Input: part model. Units: mm. Frame: model coordinates. A direction names the side the tool comes from. Coordinates: 2 decimals unless noted, no trailing zeros.
Item 1: Reachability of faces 5 (the flat face through (-62, 0, -33)), 6 (the flat face through (-70, 5, -32)) from +Z, -Z, +X, -X, +Y, -Y: full face, straight path, thin tool, end or side. Return the list, or none.
Item 2: Ray query, line 1 along X through (y, z) = (6.5, -19.5); line 2 along X through (y, z) = (7.25, -30); line 3 along Z through (x, y) = (-68.5, 9.25). Return the intervals inside material, ascending.
Item 3: Contact query for flat-ended pins moving along their axis: P1, Ø0.5, axis at x = -81.5, y = 8.5, coming from the -Z side; P2, Ø1.5, axis at y = 7, z = -29.5, coming from the -X side; P3, Ø1.5, axis at y = 2.5, z = -27.5, coming from the +X side. Output: stop coordinate, or through.
Item 4: Pull-direction query (Z, two-part tool) for faces 1 (the flat face through (-62, 10, -32)), 2 (the flat face through (-82, 9, -31.447)), 3 (the flat face through (-66.417, 8, -32)), 4 (the flat face through (-58.417, 8, -32)); classes: released by +Z, released by -Z, zero draft, split by the parting line, or undercut.
```python
from build123d import *

# Parameters (mm, degrees)
SKETCH1_R           = 20
BOSS_EXTRUDE1_DEPTH = 10
THREAD1_PITCH       = 3.175
CUT_EXTRUDE2_DEPTH  = 5


with BuildPart() as part:
    # Sketch1 → Boss-Extrude1 (new body)
    with BuildSketch(Plane(origin=(0, 0, 0), x_dir=(1, 0, 0), z_dir=(0, 1, 0))):
        with Locations(Location((-62.417227704, 31.446847546, 0), (0, 0, 270))):
            Circle(SKETCH1_R)
    extrude(amount=BOSS_EXTRUDE1_DEPTH)

    # Thread1: the profile of Thread Profile1 profile screwed along a right-hand helix of 3.149606 turns, 12 arcs to a turn; built about Z, then put on its axis
    thread1_z = Axis((0, 0, 0), (0, 0, 1))
    thread1_corners = [(20.0003, 0, -0.000173205), (20.0003, 0, 2.778298196), (18.281480847, 0, 1.785937496), (18.281480847, 0, 0.992187496)]
    with BuildLine(mode=Mode.PRIVATE) as thread1_profile:
        Line(thread1_corners[0], thread1_corners[1])
        Line(thread1_corners[1], thread1_corners[2])
        Line(thread1_corners[2], thread1_corners[3])
        Line(thread1_corners[3], thread1_corners[0])
    thread1_cap = Face(thread1_profile.wire())
    thread1_turn_angles = [0, 15, 30, 45, 60, 75, 90, 105, 120, 135, 150, 165, 180, 195, 210, 225, 240, 255, 270, 285, 300, 315, 330, 345, 360]
    thread1_turn_weights = [1, 0.9659258262890683, 1, 0.9659258262890683, 1, 0.9659258262890683, 1, 0.9659258262890683, 1, 0.9659258262890683, 1, 0.9659258262890683, 1, 0.9659258262890683, 1, 0.9659258262890683, 1, 0.9659258262890683, 1, 0.9659258262890683, 1, 0.9659258262890683, 1, 0.9659258262890683, 1]
    thread1_turn_rails = [Edge.make_bspline([Vector(p[0], p[1], 0).rotate(thread1_z, thread1_turn_angles[k]) / thread1_turn_weights[k] + Vector(0, 0, p[2] + THREAD1_PITCH * thread1_turn_angles[k] / 360) for k in range(25)], [0, 0, 0, 1, 1, 2, 2, 3, 3, 4, 4, 5, 5, 6, 6, 7, 7, 8, 8, 9, 9, 10, 10, 11, 11, 12, 12, 12], 2, thread1_turn_weights) for p in thread1_corners]
    thread1_turn_sides = [Face.make_surface_from_curves(thread1_turn_rails[p[0]], thread1_turn_rails[p[1]]) for p in [(0, 1), (1, 2), (2, 3), (3, 0)]]
    thread1_last_angles = [1080, 1095, 1110, 1121.929133858, 1133.858267717]
    thread1_last_weights = [1, 0.9659258262890683, 1, 0.9784040075425771, 1]
    thread1_last_rails = [Edge.make_bspline([Vector(p[0], p[1], 0).rotate(thread1_z, thread1_last_angles[k]) / thread1_last_weights[k] + Vector(0, 0, p[2] + THREAD1_PITCH * thread1_last_angles[k] / 360) for k in range(5)], [0, 0, 0, 1, 1, 2, 2, 2], 2, thread1_last_weights) for p in thread1_corners]
    thread1_last_sides = [Face.make_surface_from_curves(thread1_last_rails[p[0]], thread1_last_rails[p[1]]) for p in [(0, 1), (1, 2), (2, 3), (3, 0)]]
    thread1 = Plane(origin=(-62.417227704, 10, -31.446847546), x_dir=(-1, 0, 0), z_dir=(0, -1, 0)) * Solid(Shell([*[p.moved(Location((0, 0, THREAD1_PITCH * i))) for i in range(3) for p in thread1_turn_sides], *thread1_last_sides, thread1_cap, thread1_cap.rotate(thread1_z, 1133.858267717).moved(Location((0, 0, THREAD1_PITCH * 1133.858267717 / 360)))]))
    add(thread1, mode=Mode.SUBTRACT)

    # Sketch9 → Cut-Extrude2 (cut)
    with BuildSketch(Plane(origin=(0, 10, 0), x_dir=(1, 0, 0), z_dir=(0, 1, 0))):
        with BuildLine():
            Line((-66.417227704, 45.90367984), (-66.417227704, 31.446847546))
            Line((-66.417227704, 31.446847546), (-66.417227704, 16.990015251))
            add(Edge.make_bspline(
                [(-66.417227704, 45.90367984), (-88.417227704, 31.446847546), (-66.417227704, 16.990015251)],
                knots=[0, 0, 0, 1, 1, 1], degree=2))
        make_face()
        with BuildLine():
            Line((-58.417227704, 45.90367984), (-58.417227704, 16.990015251))
            add(Edge.make_bspline(
                [(-58.417227704, 45.90367984), (-36.417227704, 31.446847546), (-58.417227704, 16.990015251)],
                knots=[0, 0, 0, 1, 1, 1], degree=2))
        make_face()
    extrude(amount=-CUT_EXTRUDE2_DEPTH, mode=Mode.SUBTRACT)


solid = part.part
```
Results found:
1. face 5: +Z, -Z, +X, -X, -Y
1. face 6: +Y
2. line 1: x = -76.98 to -69.91, -66.42 to -58.42, -54.93 to -48.58
2. line 2: x = -82.36 to -77.31, -66.42 to -58.42, -47.53 to -44.19
2. line 3: z = -50.29 to -44.46, -18.43 to -12.39
3. P1: stops at z = -31.45
3. P2: stops at x = -82.38
3. P3: stops at x = -42.68
4. face 1: zero draft
4. face 2: released by -Z
4. face 3: undercut
4. face 4: undercut
